Input: part model. Units: mm. Frame: model coordinates. A direction names the side the tool comes from. Round coordinates to 2 decimals unless told otherwise and drop trailing zeros. Loops run counter-clockwise (first coordinate to the right, second up) from the corner with the lowest first, then second, coordinate; pieces in that order, holes last. Notation, with made-up numbers: (-39, -22.5) -> (14, -22.5) arc R25 ccw to (14, 0.5) -> close; hole circle Ø5 at (-12.5, 18). An arc over 180 degrees is marked (long way). One line per question, with ' | ' between items. Start each with the question number.
Q1. Cut plane A-A on x = 22. Return loops of the section in (y, z).
Q2. Material intervals for L1, parallel to X at y = 4.5, z = -33.15; L2, parallel to Z at x = -4, y = 3; L3, parallel to Y at x = -50, z = -32.85, sorted ascending.
Q3. Access query for faces 5 (the face through (25.1, 9.8, -15.861)), 6 (the face through (-50, 9.5, -34)), 7 (the face through (-4.5, 5, 23)), 8 (the face through (-50.954, 4.8, 33.521)), 9 (the face through (-45, 5, -34)). Directions: +Z, -Z, +X, -X, +Y, -Y. A direction counts if a zero-diameter tool reaches every point of the face in a straight line with its end or side. Return the directions, or none.
Q4. Cut plane C-C on y = 1.5. Return loops of the section in (x, z).
Q5. Cut plane B-B on z = 17.5. Return loops of the section in (x, y), and give its area (4 significant figures).
Q6. Contact query for flat-ended pins moving along their axis: P1, Ø3, axis at x = 21, y = 4, coming from the +Z side; P2, Ø1, axis at y = 4.5, z = 27, coming from the -X side; P3, Ø1.5, axis at x = -48, z = 33.5, coming from the +Y side; P4, Ø3, axis at x = -33, z = -2, coming from the +Y side. Output: stop coordinate, or through.
Q7. Mould query, pull axis Y, two halves, no side actions, for faces 1 (the face through (-55, -1, 0)), 2 (the face through (-50.954, 4.8, -33.479)), 3 (the face through (25, 10, 24)), 4 (the face through (-1, -2.5, 0)). Classes: pulls with the +Y half, pulls with the -Y half, needs draft (parallel to the pull), parting line crosses it, or undercut.
Q8. Cut plane D-D on x = -27. Return loops of the section in (y, z).
from build123d import *

# Parameters (mm, degrees)
SKETCH1_W             = 110
SKETCH1_H             = 70
BOSS_EXTRUDE1_DEPTH   = 2.5
SKETCH2_W             = 60
SKETCH2_H             = 12
BOSS_EXTRUDE2_DEPTH   = 1
SKETCH3_W             = 10
SKETCH3_H             = 12
BOSS_EXTRUDE3_DEPTH   = 3
SKETCH5_W             = 8
SKETCH5_H             = 9.5
BOSS_EXTRUDE4_DEPTH   = 0.5
SKETCH5_W_2           = 7
BOSS_EXTRUDE4_2_DEPTH = 0.5
SKETCH6_W             = 8
SKETCH6_H             = 9.5
SKETCH6_W_2           = 7
BOSS_EXTRUDE5_DEPTH   = 0.5
SKETCH7_W             = 60
SKETCH7_H             = 22.029201989
SKETCH7_H_2           = 19.138894139
BOSS_EXTRUDE6_DEPTH   = 0.5
CUT_EXTRUDE1_START    = -70
CUT_EXTRUDE1_DEPTH    = 70
CUT_EXTRUDE2_START    = -70
SKETCH11_R            = 1
CUT_EXTRUDE2_DEPTH    = 70
SKETCH12_W            = 13.029201989
SKETCH12_H            = 9.5
BOSS_EXTRUDE7_DEPTH   = 0.5
SKETCH13_W            = 13.029201989
SKETCH13_H            = 9.5
SKETCH13_W_2          = 11.138894139
BOSS_EXTRUDE8_DEPTH   = 0.5


with BuildPart() as part:
    # Sketch1 → Boss-Extrude1 (new body)
    with BuildSketch(Plane(origin=(0, 0, 0), x_dir=(1, 0, 0), z_dir=(0, 1, 0))):
        Rectangle(SKETCH1_W, SKETCH1_H)
    extrude(amount=-BOSS_EXTRUDE1_DEPTH)

    # Sketch2 → Boss-Extrude2 (add)
    with BuildSketch(Plane.XY.offset(35)):
        with Locations((25, 3.5)):
            Rectangle(SKETCH2_W, SKETCH2_H)
    boss_extrude2 = extrude(amount=-BOSS_EXTRUDE2_DEPTH)

    # Mirror1: Boss-Extrude2 across plane
    add(boss_extrude2.mirror(Plane.XY))

    # Sketch3 → Boss-Extrude3 (add)
    with BuildSketch(Plane.XY.offset(35)):
        with Locations((-50, 3.5)):
            Rectangle(SKETCH3_W, SKETCH3_H)
    boss_extrude3 = extrude(amount=-BOSS_EXTRUDE3_DEPTH)

    # Mirror2: Boss-Extrude3 across plane
    add(boss_extrude3.mirror(Plane.XY))

    # Sketch6 → Boss-Extrude5 (add)
    with BuildSketch(Plane.ZY.offset(5)):
        with Locations((30, 4.75)):
            Rectangle(SKETCH6_W, SKETCH6_H)
        with Locations((-30.5, 4.75)):
            Rectangle(SKETCH6_W_2, SKETCH6_H)
    extrude(amount=-BOSS_EXTRUDE5_DEPTH)



with BuildPart() as body_2:
    # Sketch5 → Boss-Extrude4 (new body)
    with BuildSketch(Plane(origin=(55, 0, 0), x_dir=(0, 0, -1), z_dir=(1, 0, 0))):
        with Locations((-30, 4.75)):
            Rectangle(SKETCH5_W, SKETCH5_H)
    extrude(amount=-BOSS_EXTRUDE4_DEPTH)


with BuildPart() as body_3:
    # Sketch5 → Boss-Extrude4 2 (new body)
    with BuildSketch(Plane(origin=(55, 0, 0), x_dir=(0, 0, -1), z_dir=(1, 0, 0))):
        with Locations((30.5, 4.75)):
            Rectangle(SKETCH5_W_2, SKETCH5_H)
    extrude(amount=-BOSS_EXTRUDE4_2_DEPTH)


with BuildPart() as part_1:
    add(part.part)

    add(body_2.part)  # Boss-Extrude6 merges body 2

    add(body_3.part)  # Boss-Extrude6 merges body 3
    # Sketch7 → Boss-Extrude6 (add)
    with BuildSketch(Plane(origin=(0, 9.5, 0), x_dir=(1, 0, 0), z_dir=(0, 1, 0))):
        with Locations((25, -23.985399005)):
            Rectangle(SKETCH7_W, SKETCH7_H)
        with Locations((25, 25.43055293)):
            Rectangle(SKETCH7_W, SKETCH7_H_2)
    extrude(amount=BOSS_EXTRUDE6_DEPTH)

    # Sketch10 → Cut-Extrude1 (cut)
    with BuildSketch(Plane(origin=(0, 0, -35), x_dir=(-1, 0, 0), z_dir=(0, 0, -1)).offset(CUT_EXTRUDE1_START)):
        with BuildLine():
            Line((0, 3.689665026), (-50, 3.689665026))
            ThreePointArc((-50, 3.689665026), (-51, 4.689665026), (-50, 5.689665026))
            Line((-50, 5.689665026), (0, 5.689665026))
            ThreePointArc((0, 5.689665026), (1, 4.689665026), (0, 3.689665026))
        make_face()
    extrude(amount=CUT_EXTRUDE1_DEPTH, mode=Mode.SUBTRACT)

    # Sketch11 → Cut-Extrude2 (cut)
    with BuildSketch(Plane(origin=(0, 0, -35), x_dir=(-1, 0, 0), z_dir=(0, 0, -1)).offset(CUT_EXTRUDE2_START)):
        with Locations((50, 4.5)):
            Circle(SKETCH11_R)
    extrude(amount=CUT_EXTRUDE2_DEPTH, mode=Mode.SUBTRACT)

    # Sketch12 → Boss-Extrude7 (add)
    with BuildSketch(Plane.ZY.offset(5)):
        Polygon((-15.861105861, 9.5), (-15.861105861, 0), (-26.92969018, 0), (-27, 9.5), align=None)
        with Locations((19.485399005, 4.75)):
            Rectangle(SKETCH12_W, SKETCH12_H)
    extrude(amount=-BOSS_EXTRUDE7_DEPTH)

    # Sketch13 → Boss-Extrude8 (add)
    with BuildSketch(Plane(origin=(55, 0, 0), x_dir=(0, 0, -1), z_dir=(1, 0, 0))):
        with Locations((-19.485399005, 4.75)):
            Rectangle(SKETCH13_W, SKETCH13_H)
        with Locations((21.43055293, 4.75)):
            Rectangle(SKETCH13_W_2, SKETCH13_H)
    extrude(amount=-BOSS_EXTRUDE8_DEPTH)


solid = part_1.part
Results:
1) outline: (-2.5, -35) -> (3.69, -35) -> (3.69, -34) -> (0, -34) -> (0, 34) -> (3.69, 34) -> (3.69, 35) -> (-2.5, 35) -> close; (5.69, -35) -> (10, -35) -> (10, -15.86) -> (9.5, -15.86) -> (9.5, -34) -> (5.69, -34) -> close; (5.69, 34) -> (9.5, 34) -> (9.5, 12.97) -> (10, 12.97) -> (10, 35) -> (5.69, 35) -> close
2) L1: -55 to -51, -49 to -45, -5 to -4.5, 54.5 to 55 | L2: -35 to -34, 34 to 35 | L3: -2.5 to 3.5, 5.5 to 9.5
3) face 5: +X, -X, +Y | face 6: +Z, -Z, -X, +Y | face 7: none | face 8: +Z, -Z | face 9: +Z, -Z, +Y
4) outline: (-55, -35) -> (-45, -35) -> (-45, -32) -> (-55, -32) -> close; (-55, 32) -> (-45, 32) -> (-45, 35) -> (-55, 35) -> close; (-5, -35) -> (55, -35) -> (55, -15.86) -> (54.5, -15.86) -> (54.5, -34) -> (-4.5, -34) -> (-4.5, -27) -> (-5, -27) -> close; (-5, -26.94) -> (-4.5, -26.94) -> (-4.5, -15.86) -> (-5, -15.86) -> close; (-5, 12.97) -> (-4.5, 12.97) -> (-4.5, 34) -> (54.5, 34) -> (54.5, 12.97) -> (55, 12.97) -> (55, 35) -> (-5, 35) -> close
5) outline: (-55, -2.5) -> (55, -2.5) -> (55, 10) -> (-5, 10) -> (-5, 0) -> (-55, 0) -> close; hole (-4.5, 0) -> (54.5, 0) -> (54.5, 9.5) -> (-4.5, 9.5) -> close | area: 314.5 mm^2
6) P1: z = 35 | P2: x = -5 | P3: y = 9.5 | P4: y = 0
7) face 1: needs draft | face 2: undercut | face 3: pulls with the +Y half | face 4: pulls with the -Y half
8) outline: (-2.5, -35) -> (0, -35) -> (0, 35) -> (-2.5, 35) -> close
